Build history of the part. All positions in model axes, mm. Face numbers are marked on the shaded views. A direction names the side the tool comes from. Give positions to 0.01 mm unless a question says otherwise; leave off trailing zeros. Write each loop counter-clockwise with the first axis right and the second up, starting at its lowest first coordinate (ties: lowest second). Pieces come first, ordered by that corner, then holes. Notation, with made-up numbers: (44, -38.5) -> (87, -38.5) arc R16 cw to (87, -34.5) -> close; hole circle Ø6 at (43, 70.5). An arc over 180 degrees is marked (long way). Put each result on its own line as item: value. Start each with the question number.
Item 1: Flat gauge pins, fed straight in: pin 1 Ø3 at (y, z) = (-84.5, -8) entering from +X; pin 2 Ø1 at (x, z) = (-11.5, -25) entering from -Y. Where does each tip first touch, or does it go through?
Item 2: Drill centre lines: line 1 along Y through (x, z) = (26, 1); line 2 along Z through (x, y) = (-2, -93.5); line 3 along X through (y, z) = (-95, 4). Where is each one in solid material? Low to high.
Item 3: Tool access for the marked faces 1 and 2: list every direction of +Z, -Z, +X, -X, +Y, -Y with a clear straight run to the whole face (end or side of a thin tool).
Item 4: Slice it at D-D, the plane y = -22.5. List the corners of the cut face in (x, z), plus the area to 3 significant figures.
Item 5: Slice it at C-C, the plane x = 0. List the corners of the cut face in (y, z), plus the area to 3 significant figures.
Item 6: Slice it at A-A, the plane y = 7. List the corners of the cut face in (x, z), plus the area to 3 significant figures.
Item 7: Slice it at B-B, the plane z = 3. List the corners of the cut face in (x, y).
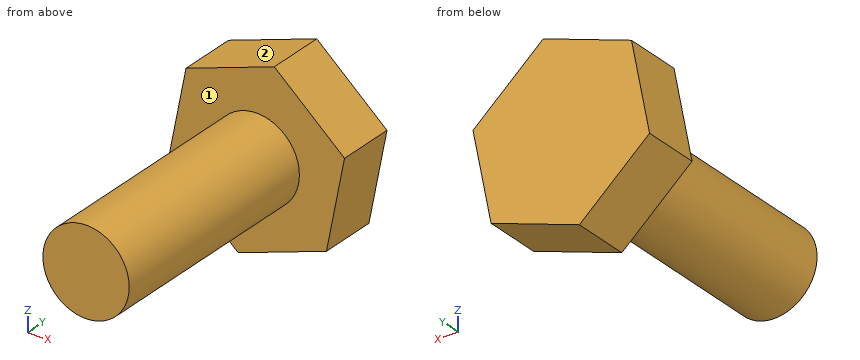
```python
from build123d import *

# Parameters (mm, degrees)
F1_DEPTH = 34.29
F2_R     = 25.531281
F3_DEPTH = 137.414
F4_R     = 11.71201
F5_DEPTH = 168.402


with BuildPart() as f1:
    # F0 (on Front) → F1 (new body)
    with BuildSketch(Plane.XZ):
        Polygon((52.237316, 17.813952), (10.691323, 54.145819), (-41.545993, 36.331867), (-52.237316, -17.813952), (-10.691323, -54.145819), (41.545993, -36.331867), align=None)
    extrude(amount=-F1_DEPTH)

    # F2 (on face) → F3 (join)
    with BuildSketch(Plane.XZ):
        Circle(F2_R)
    extrude(amount=F3_DEPTH)

    # F4 (on face) → F5 (join)
    with BuildSketch(Plane.XZ.offset(137.414)):
        Circle(F4_R)
    extrude(amount=-F5_DEPTH)


solid = f1.part
```
Values follow:
1. pin 1: x = 24.69
1. pin 2: y = 0
2. line 1: 0 to 34.29
2. line 2: -25.45 to 25.45
2. line 3: -25.22 to 25.22
3. face 1: -Y
3. face 2: +Z, -X, +Y, -Y
4. outline: circle Ø51.06 at (0, 0)
4. area: 2,050 mm2
5. outline: (-137.41, -25.53) -> (0, -25.53) -> (0, -50.5) -> (34.29, -50.5) -> (34.29, 50.5) -> (0, 50.5) -> (0, 25.53) -> (-137.41, 25.53) -> close
5. area: 10,500 mm2
6. outline: (-52.24, -17.81) -> (-10.69, -54.15) -> (41.55, -36.33) -> (52.24, 17.81) -> (10.69, 54.15) -> (-41.55, 36.33) -> close
6. area: 7,910 mm2
7. outline: (-48.13, 0) -> (-25.35, 0) -> (-25.35, -137.41) -> (25.35, -137.41) -> (25.35, 0) -> (49.31, 0) -> (49.31, 34.29) -> (-48.13, 34.29) -> close
